from build123d import *

# Parameters (mm, degrees)
EXTRUDE_1_DEPTH = 66.4
EXTRUDE_2_DEPTH = 1.5
EXTRUDE_START   = 1.5
EXTRUDE_3_DEPTH = 1.5


with BuildPart() as part:
    # 草图1 → 凸台-拉伸1 (new body)
    with BuildSketch(Plane(origin=(0, 0, 0), x_dir=(1, 0, 0), z_dir=(0, 1, 0))):
        with BuildLine():
            Line((12.55, 3.577708764), (13.55, 3.577708764))
            ThreePointArc((13.55, 3.577708764), (16.351500522, 8.675785724), (21.09000998, 12.05))
            Line((21.09000998, 12.05), (21.09000998, 13.05))
            Line((21.09000998, 13.05), (5.00999002, 13.05))
            Line((5.00999002, 13.05), (5.00999002, 12.05))
            ThreePointArc((5.00999002, 12.05), (9.748499478, 8.675785724), (12.55, 3.577708764))
        make_face()
    extrude(amount=EXTRUDE_1_DEPTH)

    # 草图2 → 凸台-拉伸2 (add)
    with BuildSketch(Plane(origin=(0, 66.4, 0), x_dir=(1, 0, 0), z_dir=(0, 1, 0))):
        with BuildLine():
            Line((5.00999002, 13.05), (5.00999002, 9.848984719))
            ThreePointArc((5.00999002, 9.848984719), (8.343981739, 7.244340463), (10.454783594, 3.577708764))
            Line((10.454783594, 3.577708764), (15.645216406, 3.577708764))
            ThreePointArc((15.645216406, 3.577708764), (17.756018261, 7.244340463), (21.09000998, 9.848984719))
            Line((21.09000998, 9.848984719), (21.09000998, 13.05))
            Line((21.09000998, 13.05), (5.00999002, 13.05))
        make_face()
    extrude(amount=EXTRUDE_2_DEPTH)

    # 草图3 → 凸台-拉伸3 (add)
    with BuildSketch(Plane.XZ.offset(EXTRUDE_START)):
        with BuildLine():
            Line((12.55, -3.577708764), (10.454783594, -3.577708764))
            ThreePointArc((10.454783594, -3.577708764), (8.343981739, -7.244340463), (5.00999002, -9.848984719))
            Line((5.00999002, -9.848984719), (5.00999002, -12.05))
            ThreePointArc((5.00999002, -12.05), (9.748499478, -8.675785724), (12.55, -3.577708764))
        make_face()
        with BuildLine():
            Line((13.55, -3.577708764), (12.55, -3.577708764))
            ThreePointArc((12.55, -3.577708764), (9.748499478, -8.675785724), (5.00999002, -12.05))
            Line((5.00999002, -12.05), (5.00999002, -13.05))
            Line((5.00999002, -13.05), (21.09000998, -13.05))
            Line((21.09000998, -13.05), (21.09000998, -12.05))
            ThreePointArc((21.09000998, -12.05), (16.351500522, -8.675785724), (13.55, -3.577708764))
        make_face()
        with BuildLine():
            Line((15.645216406, -3.577708764), (13.55, -3.577708764))
            ThreePointArc((13.55, -3.577708764), (16.351500522, -8.675785724), (21.09000998, -12.05))
            Line((21.09000998, -12.05), (21.09000998, -9.848984719))
            ThreePointArc((21.09000998, -9.848984719), (17.756018261, -7.244340463), (15.645216406, -3.577708764))
        make_face()
    extrude(amount=-EXTRUDE_3_DEPTH)


solid = part.part
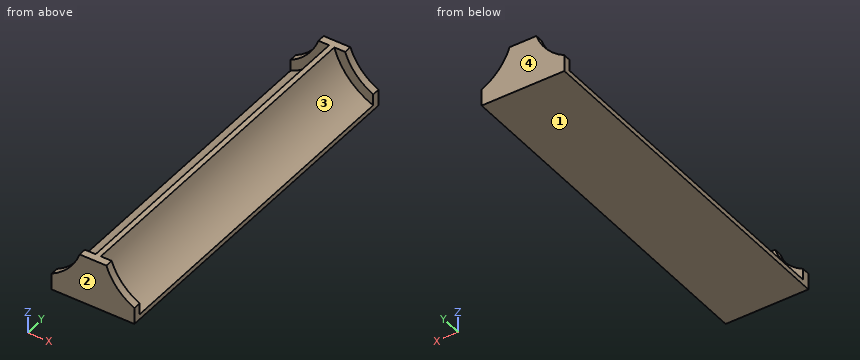
Work out the finished part from the listing and answer in its coordinate system (mm). Face numbers are marked on the shaded views. Coordinates: 2 decimals unless noted, no trailing zeros. Order: outer loops, then holes, each group sorted by start corner. A loop starts at its lowest first (then second) coordinate and runs counter-clockwise, first axis right, second up. Notation, with made-up numbers: (38, -4) - (78, -4) arc R16 ccw to (78, 22) - close; hole circle Ø11 at (-21.5, 7.5). An arc over 180 degrees is marked (long way). Put each result on its own line as item: value. Start each with the question number.
1) For a pull along Y with two mould halves and no side action, classify the marked faces 1, 2, 3 and 4 as released by +Y, released by -Y, zero draft, split by the parting line, or undercut.
2) Find section D-D (x = 8.75). Give the vertices of the cut face in (y, z).
3) Find section A-A (x = 18.5). Give the vertices of the cut face in (y, z).
4) Find section B-B (z = -6.75). Give the vertices of the cut face in (x, y), plus the area to 3 significant figures.
5) Flat-ended cylindrical pins translate along their axes: pin 1 (3 mm diameter, centred on y = 60, z = -5, fed in from -X); pin 2 (2 mm diameter, centred on y = 53.5, z = -10, fed in from -X). Find the tip coordinate at first contact, or state that the pin passes through.
6) Find the intervals of material crossed by line 1 (Y direction, x = 8.5, z = -7.25); line 2 (X direction, y = 16, z = -10.25); line 3 (Z direction, x = 15.5, y = 56), in increasing order. Write a range as from..to.
7) Find section C-C (y = 5). Give the vertices of the cut face in (x, z), plus the area to 3 significant figures.
Results list:
1. face 1: zero draft
1. face 2: released by -Y
1. face 3: undercut
1. face 4: released by +Y
2. outline: (-1.5, -13.05) - (67.9, -13.05) - (67.9, -6.75) - (66.4, -6.75) - (66.4, -9.68) - (0, -9.68) - (0, -6.75) - (-1.5, -6.75) - close
3. outline: (-1.5, -13.05) - (67.9, -13.05) - (67.9, -8.02) - (66.4, -8.02) - (66.4, -10.61) - (0, -10.61) - (0, -8.02) - (-1.5, -8.02) - close
4. outline: (8.75, -1.5) - (17.35, -1.5) - (17.35, 0) - (14.93, 0) - (14.93, 66.4) - (17.35, 66.4) - (17.35, 67.9) - (8.75, 67.9) - (8.75, 66.4) - (11.17, 66.4) - (11.17, 0) - (8.75, 0) - close
4. area: 276 mm^2
5. pin 1: stops at x = 11.32
5. pin 2: stops at x = 7.02
6. line 1: y = -1.5..0, 66.4..67.9
6. line 2: x = 8.08..18.02
6. line 3: z = -13.05..-7.61
7. outline: (5.01, -13.05) - (21.09, -13.05) - (21.09, -12.05) arc R13.05 cw to (13.55, -3.58) - (12.55, -3.58) arc R13.05 cw to (5.01, -12.05) - close
7. area: 68.6 mm^2
